Source: CAD feature listing. Evaluate the final solid. Frame: model axes, mm. A direction names the side the tool comes from. Coordinates: 2 decimals unless noted, no trailing zeros. Loops run counter-clockwise (first coordinate to the right, second up) from the corner with the lowest first, then second, coordinate; pieces in that order, holes last.
```python
from build123d import *

# Parameters (mm, degrees)
SKETCH1_R           = 7.5
BOSS_EXTRUDE1_DEPTH = 20
SKETCH1_4_W         = 22
SKETCH1_4_H         = 54
BOSS_EXTRUDE3_DEPTH = 30
CUT_EXTRUDE6_REACH  = 184.102
SKETCH5_R           = 10.5


with BuildPart() as part:
    # Sketch1 → Boss-Extrude1 (new body)
    with BuildSketch(Plane.XY):
        with BuildLine():
            Line((72.5, -57), (72.5, -12))
            Line((72.5, -12), (-72.5, -12))
            Line((-72.5, -12), (-72.5, -57))
            ThreePointArc((-72.5, -57), (-69.894587599, -66.602994193), (-62.792895003, -73.572329422))
            Line((-62.792895003, -73.572329422), (-9.292895003, -103.572329422))
            ThreePointArc((-9.292895003, -103.572329422), (0, -106), (9.292895003, -103.572329422))
            Line((9.292895003, -103.572329422), (62.792895003, -73.572329422))
            ThreePointArc((62.792895003, -73.572329422), (69.894587599, -66.602994193), (72.5, -57))
        make_face()
        with Locations((-53.5, -57)):
            Circle(SKETCH1_R, mode=Mode.SUBTRACT)
        with Locations((0, -87)):
            Circle(SKETCH1_R, mode=Mode.SUBTRACT)
        with Locations((53.5, -57)):
            Circle(SKETCH1_R, mode=Mode.SUBTRACT)
    extrude(amount=BOSS_EXTRUDE1_DEPTH)

    # Sketch1<4> → Boss-Extrude3 (add, symmetric)
    with BuildSketch(Plane.XY):
        with Locations((-61.5, 27)):
            Rectangle(SKETCH1_4_W, SKETCH1_4_H)
        with Locations((61.5, 27)):
            Rectangle(SKETCH1_4_W, SKETCH1_4_H)
        Polygon((-72.5, -12), (0, -12), (0, 0), (-50.5, 0), (-72.5, 0), align=None)
        Polygon((0, 0), (0, -12), (72.5, -12), (72.5, 0), (50.5, 0), align=None)
    extrude(amount=BOSS_EXTRUDE3_DEPTH, both=True)

    # Cut-Extrude6: up to this face of the body (flat: up to its plane)
    cut_extrude6_end = Plane(part.part.faces().sort_by_distance((-72.5, 10.722222222, 1.851851852))[0])
    # Sketch5 → Cut-Extrude6 (cut, up to the picked face)
    with BuildSketch(Plane(origin=(72.5, 0, 0), x_dir=(0, 0, -1), z_dir=(1, 0, 0)), mode=Mode.PRIVATE) as cut_extrude6_sk1:
        with BuildLine():
            Line((-13, -12), (-13, 21))
            ThreePointArc((-13, 21), (8, 42), (29, 21))
            Line((29, 21), (29, -12))
            Line((29, -12), (30, -12))
            Line((30, -12), (30, 54))
            Line((30, 54), (-30, 54))
            Line((-30, 54), (-30, -12))
            Line((-30, -12), (-20, -12))
            Line((-20, -12), (-13, -12))
        make_face()
    cut_extrude6_tool1 = split(extrude(cut_extrude6_sk1.sketch, amount=-CUT_EXTRUDE6_REACH, mode=Mode.PRIVATE), bisect_by=cut_extrude6_end, keep=Keep.BOTH, mode=Mode.PRIVATE)
    # Sketch5 → Cut-Extrude6 (cut, up to the picked face)
    with BuildSketch(Plane(origin=(72.5, 0, 0), x_dir=(0, 0, -1), z_dir=(1, 0, 0)), mode=Mode.PRIVATE) as cut_extrude6_sk2:
        with Locations((8, 21)):
            Circle(SKETCH5_R)
    cut_extrude6_tool2 = split(extrude(cut_extrude6_sk2.sketch, amount=-CUT_EXTRUDE6_REACH, mode=Mode.PRIVATE), bisect_by=cut_extrude6_end, keep=Keep.BOTH, mode=Mode.PRIVATE)
    add(cut_extrude6_tool1.solids().sort_by(Axis((72.5, 4.5, 13.891964), (-1, 0, 0)))[0], mode=Mode.SUBTRACT)
    add(cut_extrude6_tool2.solids().sort_by(Axis((72.5, 21, -8), (-1, 0, 0)))[0], mode=Mode.SUBTRACT)


solid = part.part
```
Q1. Reachability of faces 1 (the flat face through (-1, -48, 0)), 2 (the flat face through (1, -3, 13)), 3 (the cylindrical face through (61.65, 31.41, -6.63)) from +Z, -Z, +X, -X, +Y, -Y: full face, straight path, thin tool, end or side. Return the list, or none.
Q2. Section query C-C on y = -91. Return the cut outline in (x, z), then the cut area to 3 significant figures.
Q3. Section query D-D on y = 23.5. Return the cut outline in (x, z).
Q4. First-contact query: pin 1 Ø12.5 at (y, z) = (24, -12.5) entering from -X; pin 2 Ø6 at (x, z) = (-34.5, -21) entering from +Y; pin 3 Ø3.5 at (x, z) = (24.5, 15.5) entering from +Y; pin 4 Ø2 at (x, z) = (-48.5, -8.5) entering from -Y. Flat tips, straight axial feed; report the tip coordinate or a pass-through.
Q5. Section query A-A on x = -53.5. Return the cut outline in (y, z).
Q6. Section query B-B on x = 0. Return the cut outline in (y, z), then the cut area to 3 significant figures.
Q7. Draft query along Y for faces 4 (the flat face through (1, -12, 17)), 5 (the cylindrical face through (-54.476, -49.564, 9.86)), 6 (the cylindrical face through (0, -106, 10)), 7 (the flat face through (-50.5, 11, -3)). Return one class per face: released by +Y, released by -Y, zero draft, split by the parting line, or undercut.
Q8. Material intervals for line 1 along Y through (x, z) = (-64.75, -8); line 2 along Y through (x, z) = (0, 6.75); line 3 along X through (y, z) = (-62, 15), sorted ascending.
Resolved:
1. face 1: -Z, +X, -X, -Y
1. face 2: +Z, +X, -X, +Y
1. face 3: +X, -X
2. outline: (-31.71, 0) - (-6.34, 0) - (-6.34, 20) - (-31.71, 20) - close; (6.34, 0) - (31.71, 0) - (31.71, 20) - (6.34, 20) - close
2. area: 1,010 mm2
3. outline: (-72.5, -28.85) - (-50.5, -28.85) - (-50.5, -18.2) - (-72.5, -18.2) - close; (-72.5, 2.2) - (-50.5, 2.2) - (-50.5, 12.85) - (-72.5, 12.85) - close; (50.5, -28.85) - (72.5, -28.85) - (72.5, -18.2) - (50.5, -18.2) - close; (50.5, 2.2) - (72.5, 2.2) - (72.5, 12.85) - (50.5, 12.85) - close
4. pin 1: stops at x = -72.5
4. pin 2: stops at y = 0
4. pin 3: stops at y = -12
4. pin 4: stops at y = -12
5. outline: (-78.78, 0) - (-64.5, 0) - (-64.5, 20) - (-78.78, 20) - close; (-49.5, 0) - (-12, 0) - (-12, -29) - (21, -29) arc R21 ccw to (21, 13) - (-12, 13) - (-12, 20) - (-49.5, 20) - close; hole circle Ø21 at (21, -8)
6. outline: (-106, 0) - (-94.5, 0) - (-94.5, 20) - (-106, 20) - close; (-79.5, 0) - (-12, 0) - (-12, -29) - (0, -29) - (0, 13) - (-12, 13) - (-12, 20) - (-79.5, 20) - close
6. area: 2,080 mm2
7. face 4: released by +Y
7. face 5: undercut
7. face 6: released by -Y
7. face 7: zero draft
8. line 1: y = -12 to 10.5, 31.5 to 42
8. line 2: y = -106 to -94.5, -79.5 to 0
8. line 3: x = -71.83 to -59.09, -47.91 to 47.91, 59.09 to 71.83
